Check sheet for the modelled part. Datum: model origin and axes. Units: mm. Face numbers are marked on the shaded views. Coordinates: 2 decimals unless noted, no trailing zeros. Loops run counter-clockwise (first coordinate to the right, second up) from the corner with the lowest first, then second, coordinate; pieces in that order, holes last. Notation, with made-up numbers: M 16.25,-19 L 62.25,-19 A25 cw 62.25,3 Z; hole C 57.25,13.5 d10. An arc over 180 degrees is marked long. Return JSON: item names as keys, results as strings.
Autodesk Inventor part; units mm, degrees
ref_plane "YZ Plane" through (0, 0, 0) normal (1, 0, 0) x (0, 1, 0)
ref_plane "XZ Plane" through (0, 0, 0) normal (0, 1, 0) x (-1, 0, 0)
ref_plane "XY Plane" through (0, 0, 0) normal (0, 0, 1) x (1, 0, 0)
sketch "Szkic1" plane through (0, 0, 0) normal (0, 0, 1) x (1, 0, 0)
  circle A0 centre (0, 0) radius 15
  circle A1 centre (0, 0) radius 13
  dimension "d0" = 30
  dimension "d2" = 2
extrude "Wyciągnięcie proste1" add sketch "Szkic1" along normal mid plane 125
sketch "Szkic5" plane through (0, 0, 0) normal (0, 1, 0) x (-1, 0, 0)
  circle A0 centre (0, 55) radius 1.5
  circle A1 centre (0, -55) radius 1.5
  point P0 (0, 0)
  dimension "d40" = 3
  dimension "d41" = 3
extrude "Wyciągnięcie proste6" cut sketch "Szkic5" against normal blind 20
sketch "Szkic6" plane through (0, 0, 0) normal (1, 0, 0) x (0, 1, 0)
  circle A0 centre (0, 55) radius 4
  point P0 (0, 0)
  dimension "d44" = 8
extrude "Wyciągnięcie proste7" cut sketch "Szkic6" along normal mid plane 30
properties part number "rura_30_2_250" material "Aluminium 6061"
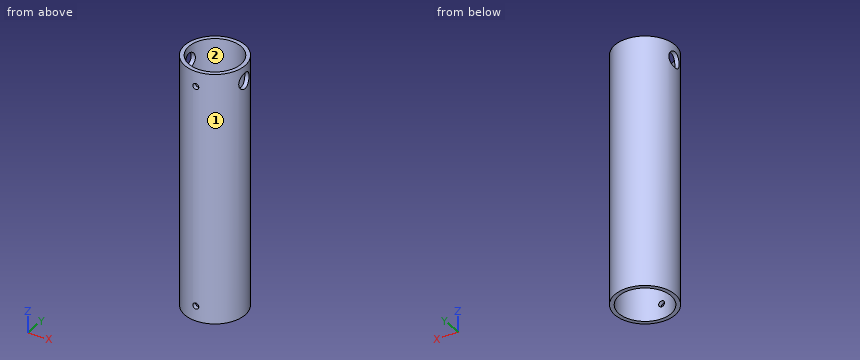
1) Draft check along Y on the marked faces 1 and 2. Enter one of: +Y half, -Y half, draft (parallel to the pull), parting line (faces both ways), or undercut.
Answers:
{"face 1": "parting line", "face 2": "undercut"}
2) Section check A-A on x = 0. Record the cut outline in (y, z).
Answers:
{"outline": "M -15,-62.5 L -13,-62.5 L -13,-56.5 L -15,-56.5 Z; M -15,-53.5 L -13,-53.5 L -13,53.5 L -15,53.5 Z; M -15,56.5 L -13,56.5 L -13,62.5 L -15,62.5 Z; M 13,-62.5 L 15,-62.5 L 15,62.5 L 13,62.5 Z"}
3) Go/stop test with flat-tipped pins: pin 1 Ø6.5 at (y, z) = (0, 55) entering from -X; pin 2 Ø3 at (y, z) = (-9, 28.5) entering from -X; pin 3 Ø12 at (x, z) = (-8.5, 44) entering from +Y; pin 4 Ø1.8 at (x, z) = (0, 55) entering from -Y. Record where each tip stops, or that it passes through.
Answers:
{"pin 1": "through", "pin 2": "x = -12.99", "pin 3": "y = 14.79", "pin 4": "y = 12.97"}
4) Section check C-C on z = 55. Record the cut outline in (x, y).
Answers:
{"outline": "M -14.46,-4 A15 ccw -1.5,-14.92 L -1.5,-12.91 A13 cw -12.37,-4 Z; M -14.46,4 L -12.37,4 A13 cw 12.37,4 L 14.46,4 A15 ccw Z; M 1.5,-14.92 A15 ccw 14.46,-4 L 12.37,-4 A13 cw 1.5,-12.91 Z"}
5) Scan lines: line 1 along Z through (x, y) = (14, 0); line 2 along Y through (x, z) = (0, -19). Record each from-to range of solid material in increasing order. Write a range as [from, to].
Answers:
{"line 1": "[-62.5, 51], [59, 62.5]", "line 2": "[-15, -13], [13, 15]"}
6) Section check B-B on y = 0. Record the cut outline in (x, z), then the cut area to 3 significant figures.
Answers:
{"outline": "M -15,-62.5 L -13,-62.5 L -13,51 L -15,51 Z; M -15,59 L -13,59 L -13,62.5 L -15,62.5 Z; M 13,-62.5 L 15,-62.5 L 15,51 L 13,51 Z; M 13,59 L 15,59 L 15,62.5 L 13,62.5 Z", "area": "468 mm²"}
7) Section check D-D on x = 5. Record the cut outline in (y, z).
Answers:
{"outline": "M -14.14,-62.5 L -12,-62.5 L -12,62.5 L -14.14,62.5 Z; M 12,-62.5 L 14.14,-62.5 L 14.14,62.5 L 12,62.5 Z"}
